CAD build for the part. Positions are in the model's coordinates, mm. Face numbers are marked on the shaded views. A direction names the side the tool comes from. Round coordinates to 2 decimals unless told otherwise and drop trailing zeros. Write each loop counter-clockwise with the first axis right and the second up, starting at its lowest first coordinate (ties: lowest second). Pieces come first, ordered by that corner, then holes. Notation, with made-up numbers: (61, 71) -> (108, 71) arc R29 ccw to (108, 105) -> close; hole circle Ø10 at (66, 80). An arc over 180 degrees is marked (long way). Answer in a Markdown table with one row per item. Add a question column.
Autodesk Fusion 360 part; units mm, degrees
sketch "Sketch1" plane through (0, 0, 0) normal (0, 0, 1) x (1, 0, 0) in component "Servohalterung"
  line L0 (0, 0) -> (58, 0)
  line L1 (58, 0) -> (58, 29)
  line L2 (58, 29) -> (0, 29)
  line L3 (0, 29) -> (0, 0)
  line L4 (8, 27) -> (50, 27)
  line L5 (50, 27) -> (50, 6)
  line L6 (50, 6) -> (8, 6)
  line L7 (8, 6) -> (8, 27)
  dimension "d22" = 8
  dimension "d23" = 8
  dimension "d24" = 42
  dimension "d25" = 2
  dimension "d26" = 6
  dimension "d27" = 21
extrude "Extrude1" add sketch "Sketch1" along normal blind 6 in component "Servohalterung"
sketch "Sketch2" plane through (0, 0, 6) normal (0, 0, 1) x (-1, 0, 0) in component "Servohalterung"
  line L0 (-50, -6) -> (-8, -6)
  line L1 (-8, -6) -> (-8, -27)
  line L2 (-8, -27) -> (-50, -27)
  line L3 (-50, -27) -> (-50, -6)
  line L4 (0, -29) -> (0, 0)
  line L5 (0, 0) -> (-58, 0)
  line L6 (-58, 0) -> (-58, -29)
  line L7 (-58, -29) -> (0, -29)
  line L8 (0, 0) -> (-58, 0)
  line L9 (-58, 0) -> (-58, -6)
  line L10 (-58, -6) -> (0, -6)
  line L11 (0, -6) -> (0, 0)
  line L12 (-50, -6) -> (-8, -6)
extrude "Extrude2" add sketch "Sketch2" along normal blind 14 contours L0 L4 L5 L6 L8 L9 L10 L11 L12 in component "Servohalterung"
sketch "Sketch3" plane through (0, 6, 0) normal (0, 1, 0) x (-1, 0, 0) in component "Servohalterung"
  line L0 (-8, 0) -> (-8, 6)
  line L1 (-8, 6) -> (0, 6)
  line L2 (0, 6) -> (0, 20)
  line L3 (0, 20) -> (-58, 20)
  line L4 (-58, 20) -> (-58, 6)
  line L5 (-58, 6) -> (-50, 6)
  line L6 (-50, 6) -> (-50, 0)
  line L7 (-50, 0) -> (-8, 0)
  circle A0 centre (-40, 10) radius 6
  line L8 (-29, 0) -> (-29, 20)
  circle A1 centre (-18, 10) radius 6
  dimension "d34" = 12
  dimension "d38" = 10
  dimension "d64" = 10
extrude "Extrude3" cut sketch "Sketch3" against normal blind 4 contours A0 | A1 in component "Servohalterung"
sketch "Sketch4" plane through (0, 2, 0) normal (0, 1, 0) x (-1, 0, 0) in component "Servohalterung"
  circle A0 centre (-40, 10) radius 6
  circle A1 centre (-40, 10) radius 2.75
  line L0 (-28.3646, -4) -> (-28.3646, 24)
  circle A2 centre (-18, 10) radius 2.75
  circle A3 centre (-18, 10) radius 6
  line L1 (-58, 20) -> (0, 20)
  dimension "d42" = 5.5
  dimension "d43" = 5.5
extrude "Extrude4" cut sketch "Sketch4" against normal up to surface (2 mm away) contours A1 | A2 in component "Servohalterung"
sketch "Sketch5" plane through (0, 0, 6) normal (0, 0, 1) x (-1, 0, 0) in component "Servohalterung"
  line L0 (0, -6) -> (-8, -6)
  line L1 (-8, -6) -> (-8, -27)
  line L2 (-8, -27) -> (-50, -27)
  line L3 (-50, -27) -> (-50, -6)
  line L4 (-50, -6) -> (-58, -6)
  line L5 (-58, -6) -> (-58, -29)
  line L6 (-58, -29) -> (0, -29)
  line L7 (0, -29) -> (0, -6)
  circle A0 centre (-4.5, -22.3) radius 2.5
  circle A1 centre (-4.5, -12.3) radius 2.5
  circle A2 centre (-53.5, -22.3) radius 2.5
  circle A3 centre (-53.5, -12.3) radius 2.5
  dimension "d46" = 5
  dimension "d48" = 2.2
  dimension "d49" = 1
  dimension "d50" = 5
  dimension "d51" = 5
  dimension "d52" = 5
  dimension "d53" = 5
  dimension "d54" = 5
  dimension "d57" = 1
extrude "Extrude5" cut sketch "Sketch5" against normal up to surface (6 mm away) contours A0 | A1 | A2 | A3 in component "Servohalterung"
chamfer "Chamfer3" distance 3 angle 45 2 edges at (58, 29, 3) (0, 29, 3) in component "Servohalterung"
chamfer "Chamfer1" distance 1 angle 45 12 edges at (58, 13, 0) (58, 16, 6) (29, 29, 6) (29, 29, 0) (0, 13, 0) (0, 16, 6) (1.5, 27.5, 0) (1.5, 27.5, 6) (56.5, 27.5, 0) (56.5, 27.5, 6) (0, 6, 13) (58, 6, 13) in component "Servohalterung"
component "Servohalterung" placed x (1, 0, 0) y (0, 1, 0) z (0, 0, 1) at (0, 0, 0)
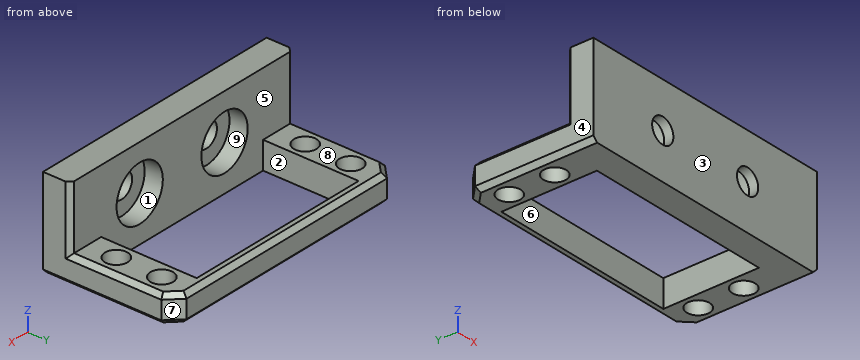
Item 1: Saw through at D-D on y = 12.3. Give the cut face in (x, z), then the cut area to 3 significant figures.
Item 2: Saw through at C-C on y = 7. Give the cut face in (x, z).
Item 3: Pin check, flat tips, straight feed: pin 1 (6 mm diameter, centred on x = 53.5, y = 12.3, fed in from +Z); pin 2 (6.5 mm diameter, centred on x = 18, z = 10, fed in from +Y); pin 3 (1.5 mm diameter, centred on x = 30, z = 7, fed in from +Y). Stop position of each tip, or through.
Item 4: Drill centre lines: probe 1 along Y at (x, z) = (53.5, 1.7); probe 2 along X at (y, z) = (22.3, 3.05); probe 3 along Z at (x, y) = (40, 3.4). Where is each one in solid material? Low to high.
Item 5: Saw through at A-A on x = 18. Give the cut face in (y, z), then the cut area to 3 significant figures.
Item 6: Two-plate mould, pull along Y, no slides. Class the marked faces 1, 2, 3 and 4: +Y half, -Y half, draft (parallel to the pull), parting line (faces both ways), or undercut.
Item 7: Saw through at B-B on z = 10. Give the cut face in (x, y), then the cut area to 3 significant figures.
Item 8: Tool access for the marked faces 5, 6, 7, 8 and 9: list every direction of +Z, -Z, +X, -X, +Y, -Y with a clear straight run to the whole face (end or side of a thin tool).
Recorded:
| question | item | result |
|---|---|---|
| 1 | outline | (0, 1) -> (1, 0) -> (2, 0) -> (2, 6) -> (1, 6) -> (0, 5) -> close; (7, 0) -> (8, 0) -> (8, 6) -> (7, 6) -> close; (50, 0) -> (51, 0) -> (51, 6) -> (50, 6) -> close; (56, 0) -> (57, 0) -> (58, 1) -> (58, 5) -> (57, 6) -> (56, 6) -> close |
| 1 | area | 34.0 mm2 |
| 2 | outline | (0, 1) -> (1, 0) -> (8, 0) -> (8, 6) -> (1, 6) -> (0, 5) -> close; (50, 0) -> (57, 0) -> (58, 1) -> (58, 5) -> (57, 6) -> (50, 6) -> close |
| 3 | pin 1 | z = 6 |
| 3 | pin 2 | y = 2 |
| 3 | pin 3 | y = 6 |
| 4 | probe 1 | 0 to 9.8, 14.8 to 19.8, 24.8 to 29 |
| 4 | probe 2 | 0 to 2, 7 to 8, 50 to 51, 56 to 58 |
| 4 | probe 3 | 0 to 4, 16 to 20 |
| 5 | outline | (0, 0) -> (6, 0) -> (6, 4) -> (2, 4) -> (2, 7.25) -> (0, 7.25) -> close; (0, 12.75) -> (2, 12.75) -> (2, 16) -> (6, 16) -> (6, 20) -> (0, 20) -> close; (27, 0) -> (28, 0) -> (29, 1) -> (29, 5) -> (28, 6) -> (27, 6) -> close |
| 5 | area | 72.0 mm2 |
| 6 | face 1 | undercut |
| 6 | face 2 | undercut |
| 6 | face 3 | -Y half |
| 6 | face 4 | draft |
| 7 | outline | (0, 0) -> (15.25, 0) -> (15.25, 2) -> (12, 2) -> (12, 6) -> (1, 6) -> (0, 5) -> close; (20.75, 0) -> (37.25, 0) -> (37.25, 2) -> (34, 2) -> (34, 6) -> (24, 6) -> (24, 2) -> (20.75, 2) -> close; (42.75, 0) -> (58, 0) -> (58, 5) -> (57, 6) -> (46, 6) -> (46, 2) -> (42.75, 2) -> close |
| 7 | area | 229 mm2 |
| 8 | face 5 | +Z |
| 8 | face 6 | +Z, -Z |
| 8 | face 7 | +Z, -Z, +X, +Y |
| 8 | face 8 | +Z, +X, -X, +Y |
| 8 | face 9 | none |
